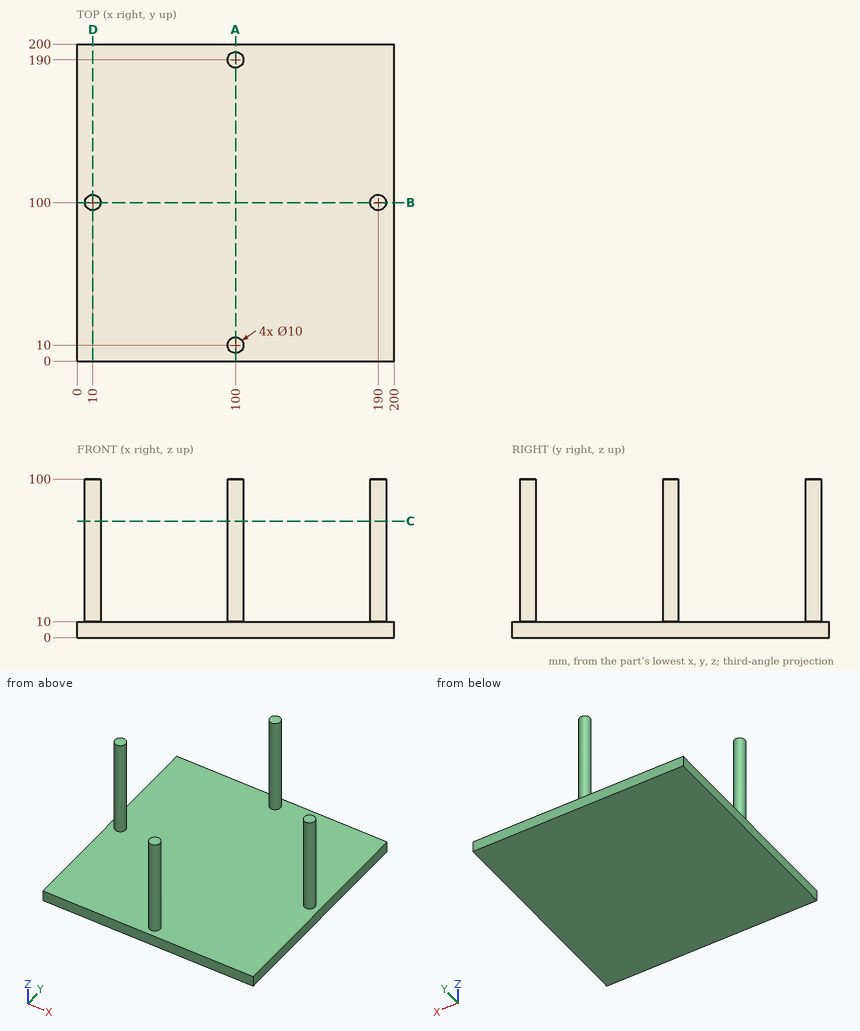
Part print with two shaded views. Sizes in mm from the minimum x, y, z corner. Coordinates: 2 decimals unless noted, no trailing zeros. Write each loop counter-clockwise with the first axis right and the second up, starting at its lowest first coordinate (ties: lowest second). Pieces come first, ordered by that corner, then holes. Notation, with made-up numbers: (69, 29.5) - (95, 29.5) arc R35 ccw to (95, 66.5) - close; hole circle Ø2 at (-5, 89). An arc over 180 degrees is marked (long way). Put each result on its own line as item: value.
1. Band-saw the part on A-A (x = 100). Write the cut outline in (y, z).
Final values:
outline: (0, 0) - (200, 0) - (200, 10) - (195, 10) - (195, 100) - (185, 100) - (185, 10) - (15, 10) - (15, 100) - (5, 100) - (5, 10) - (0, 10) - close
2. Band-saw the part on C-C (z = 73.5). Write the cut outline in (x, y), then the cut area to 3 significant figures.
Final values:
outline: circle Ø10 at (10, 100); circle Ø10 at (100, 10); circle Ø10 at (100, 190); circle Ø10 at (190, 100)
area: 314 mm²
3. Probe line 1 along Y through (x, z) = (100.5, 44); line 2 along Z through (x, y) = (178, 52); line 3 along X through (y, z) = (99, 60.5). List the from-to ranges inside material, lowest first. Write a range as [from, to].
Final values:
line 1: y = [5.03, 14.97], [185.03, 194.97]
line 2: z = [0, 10]
line 3: x = [5.1, 14.9], [185.1, 194.9]
4. Flat gauge pins, fed straight in: pin 1 Ø3 at (x, z) = (105, 73) entering from -Y; pin 2 Ø1.5 at (x, y) = (44, 155.5) entering from +Z. Where does each tip first touch, or does it go through?
Final values:
pin 1: stops at y = 6.43
pin 2: stops at z = 10
5. Band-saw the part on D-D (x = 10). Write the cut outline in (y, z).
Final values:
outline: (0, 0) - (200, 0) - (200, 10) - (105, 10) - (105, 100) - (95, 100) - (95, 10) - (0, 10) - close
